Here's the drawing with two shaded views (mm, measured from the low corner). I have some questions. A direction names the side the tool comes from. Coordinates: 2 decimals unless noted, no trailing zeros. Write each loop counter-clockwise with the first axis right and the second up, starting at its lowest first coordinate (ties: lowest second). Pieces come first, ordered by that corner, then holes.
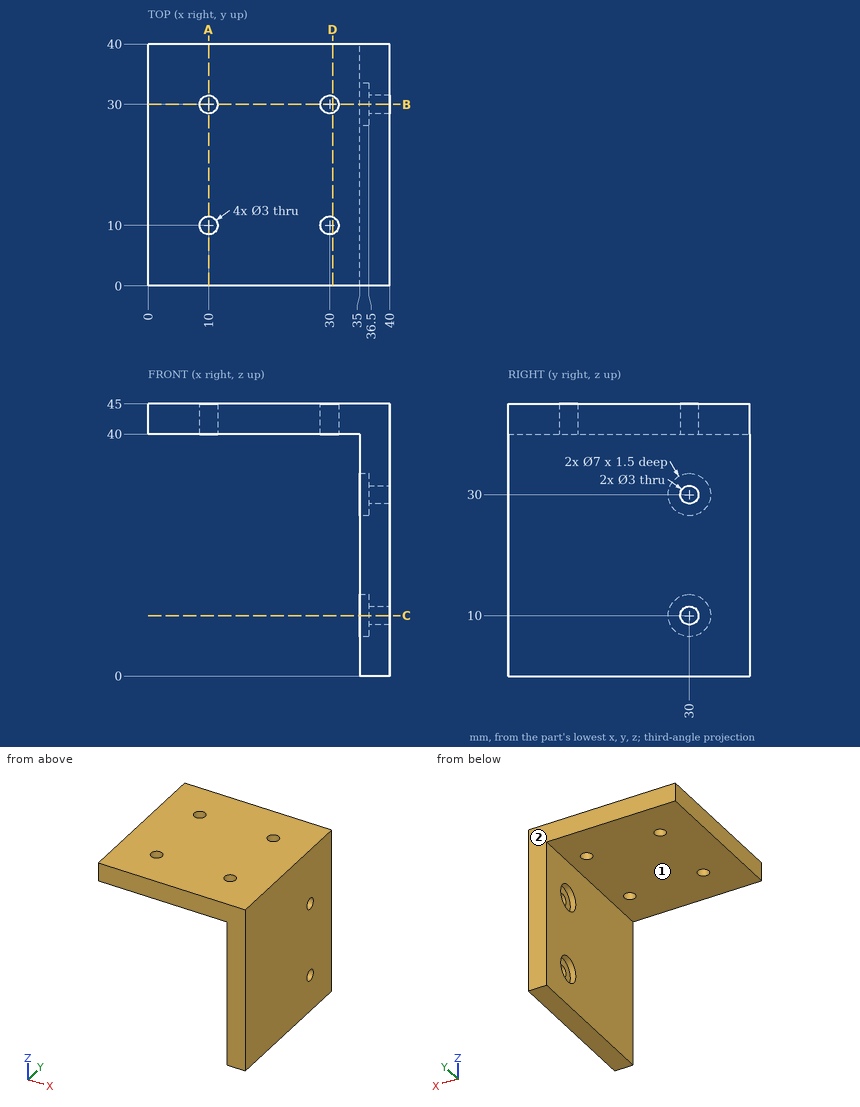
1. For pin 1 (4 mm diameter, centred on y = 30, z = 10, fed in from -X); pin 2 (4 mm diameter, centred on x = 9.5, y = 14.5, fed in from -Z); pin 3 (2.5 mm diameter, centred on x = 30, y = 30, fed in from -Z); pin 4 (5.5 mm diameter, centred on y = 28.5, z = 29.5, fed in from -X), each with a flat end and sliding along its axis, tell me the tip position at first contact or that it passes through.
Verdict:
pin 1: stops at x = 36.5
pin 2: stops at z = 40
pin 3: passes through
pin 4: stops at x = 35
2. I want a section at C-C on z = 10. Please give me the cut outline in (x, y).
Verdict:
outline: (35, 0) - (40, 0) - (40, 28.5) - (36.5, 28.5) - (36.5, 26.5) - (35, 26.5) - close; (35, 33.5) - (36.5, 33.5) - (36.5, 31.5) - (40, 31.5) - (40, 40) - (35, 40) - close
3. Please list where these lines run through material, in increasing order: line 1 along Y through (x, z) = (30, 43.4); line 2 along Y through (x, z) = (35.5, 30); line 3 along Y through (x, z) = (37.9, 10).
Verdict:
line 1: y = 0 to 8.5, 11.5 to 28.5, 31.5 to 40
line 2: y = 0 to 26.5, 33.5 to 40
line 3: y = 0 to 28.5, 31.5 to 40
4. I want a section at B-B on y = 30. Give the number of separate pieces and of enclosed holes in the cut face, plus the area to 3 significant figures.
Verdict:
separate pieces: 5
enclosed holes: 0
area: 328 mm2
5. On a 3-axis mill with a long thin cutter (end or side, diameter ignored), from which of +Z, -Z, +X, -X, +Y, -Y can I reach the whole of each face in a straight line? I mean the marked faces 1 and 2. Say none if no direction works.
Verdict:
face 1: -Z, -X, +Y, -Y
face 2: +Z, -Z, +X, -X, +Y
6. I want a section at D-D on x = 30.5. Please give me the cut outline in (y, z).
Verdict:
outline: (0, 40) - (8.59, 40) - (8.59, 45) - (0, 45) - close; (11.41, 40) - (28.59, 40) - (28.59, 45) - (11.41, 45) - close; (31.41, 40) - (40, 40) - (40, 45) - (31.41, 45) - close
7. I want a section at A-A on x = 10. Please give me the cut outline in (y, z).
Verdict:
outline: (0, 40) - (8.5, 40) - (8.5, 45) - (0, 45) - close; (11.5, 40) - (28.5, 40) - (28.5, 45) - (11.5, 45) - close; (31.5, 40) - (40, 40) - (40, 45) - (31.5, 45) - close
